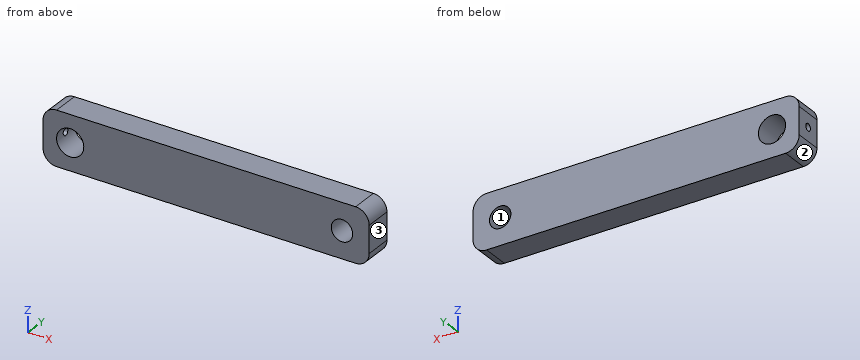
from build123d import *

# Parameters (mm, degrees)
SKETCH1_W                        = 152.4
SKETCH1_H                        = 25.4
SKETCH1_R                        = 6.35
SKETCH1_R_2                      = 5
BOSS_EXTRUDE1_DEPTH              = 12.7
FILLET1_R                        = 6.35
TAP_DRILL_FOR_M4X0_7_TAP1_REACH  = 155.455
TAP_DRILL_FOR_M4X0_7_TAP1_BORE_R = 1.65


with BuildPart() as part:
    # Sketch1 → Boss-Extrude1 (new body)
    with BuildSketch(Plane(origin=(0, 0, 0), x_dir=(1, 0, 0), z_dir=(0, 1, 0))):
        with Locations((63.5, 0)):
            Rectangle(SKETCH1_W, SKETCH1_H)
        with Locations(Location((0, 0, 0), (0, 0, 270))):
            Circle(SKETCH1_R, mode=Mode.SUBTRACT)
        with Locations(Location((127, 0, 0), (0, 0, 270))):
            Circle(SKETCH1_R_2, mode=Mode.SUBTRACT)
    extrude(amount=BOSS_EXTRUDE1_DEPTH)

    # Fillet1
    fillet1_edges = [part.edges().sort_by_distance(p)[0] for p in [
        (-12.7, 6.35, -12.7),
        (139.7, 6.35, -12.7),
        (139.7, 6.35, 12.7),
        (-12.7, 6.35, 12.7),
    ]]
    fillet(fillet1_edges, radius=FILLET1_R)

    # Tap Drill for M4x0.7 Tap1 bore → Tap Drill for M4x0.7 Tap1 (cut, up to next)
    with BuildSketch(Plane.ZY.offset(12.7), mode=Mode.PRIVATE) as tap_drill_for_m4x0_7_tap1_sk1:
        with Locations((0, 6.35)):
            Circle(TAP_DRILL_FOR_M4X0_7_TAP1_BORE_R)
    tap_drill_for_m4x0_7_tap1_tool1 = extrude(tap_drill_for_m4x0_7_tap1_sk1.sketch, amount=-TAP_DRILL_FOR_M4X0_7_TAP1_REACH, mode=Mode.PRIVATE) & part.part
    add(tap_drill_for_m4x0_7_tap1_tool1.solids().sort_by_distance((-12.7, 6.35, 0))[0], mode=Mode.SUBTRACT)


solid = part.part
Can you work these out from the model? Positions are in its coordinate system, mm. Face numbers are marked on the shaded views. Round coordinates to 2 decimals unless told otherwise and drop trailing zeros. Write each loop counter-clockwise with the first axis right and the second up, starting at its lowest first coordinate (ties: lowest second). Pieces come first, ordered by that corner, then holes. Notation, with made-up numbers: M 40,83.5 L 66,83.5 A24 ccw 66,114.5 Z; hole C 63.25,88.5 d10. An arc over 180 degrees is marked long. Use a Markdown table: item, result.
Item 1: If I drill on line 1 along X through (y, z) = (4, 0); line 2 along X through (y, z) = (11.5, -3.5); line 3 along Y through (x, z) = (-10.25, 0), over which ranges is the centre line in solid material (lowest first)? Write a range as [from, to].
Found:
| item | result |
|---|---|
| line 1 | x = [-12.7, -6.35], [6.35, 122], [132, 139.7] |
| line 2 | x = [-12.7, -5.3], [5.3, 123.43], [130.57, 139.7] |
| line 3 | y = [0, 4.7], [8, 12.7] |
Item 2: I want a section at B-B (z = 0). List the corners of the cut face in (x, y) for me.
Found:
| item | result |
|---|---|
| outline | M -12.7,0 L -6.35,0 L -6.35,4.7 L -12.7,4.7 Z; M -12.7,8 L -6.35,8 L -6.35,12.7 L -12.7,12.7 Z; M 6.35,0 L 122,0 L 122,12.7 L 6.35,12.7 Z; M 132,0 L 139.7,0 L 139.7,12.7 L 132,12.7 Z |
Item 3: We'd pull the mould along X, two halves only. Please class the marked faces 1, 2 and 3: released by +X, released by -X, zero draft, split by the parting line, or undercut.
Found:
| item | result |
|---|---|
| face 1 | undercut |
| face 2 | released by -X |
| face 3 | released by +X |
Item 4: I want a section at D-D (x = 127). List the corners of the cut face in (y, z) for me.
Found:
| item | result |
|---|---|
| outline | M 0,-12.7 L 12.7,-12.7 L 12.7,-5 L 0,-5 Z; M 0,5 L 12.7,5 L 12.7,12.7 L 0,12.7 Z |
Item 5: I want a section at A-A (y = 3). List the corners of the cut face in (x, z) for me, and give its area (3 significant figures).
Found:
| item | result |
|---|---|
| outline | M -12.7,-6.35 A6.35 ccw -6.35,-12.7 L 133.35,-12.7 A6.35 ccw 139.7,-6.35 L 139.7,6.35 A6.35 ccw 133.35,12.7 L -6.35,12.7 A6.35 ccw -12.7,6.35 Z; hole C 0,0 d12.7; hole C 127,0 d10 |
| area | 3,630 mm2 |
Item 6: I want a section at C-C (x = 0). List the corners of the cut face in (y, z) for me, and give its area (3 significant figures).
Found:
| item | result |
|---|---|
| outline | M 0,-12.7 L 12.7,-12.7 L 12.7,-6.35 L 0,-6.35 Z; M 0,6.35 L 12.7,6.35 L 12.7,12.7 L 0,12.7 Z |
| area | 161 mm2 |
